Verification items for the finished model (mm, model axes). A direction names the side the tool comes from. Round coordinates to 2 decimals unless told otherwise and drop trailing zeros. Write each loop counter-clockwise with the first axis right and the second up, starting at its lowest first coordinate (ties: lowest second). Pieces come first, ordered by that corner, then holes. Notation, with made-up numbers: (20, -6.5) - (50, -6.5) arc R20 ccw to (50, 21.5) - close; hole circle Ø8 at (67.5, 46). An arc over 180 degrees is marked (long way). Answer as a JSON object with one key per item and string values.
```python
from build123d import *

# Parameters (mm, degrees)
SKETCH2_R                       = 24.765
BOSS_EXTRUDE1_DEPTH             = 10.16
CHAMFER1_SIZE                   = 2.54
CHAMFER2_SIZE                   = 0.254
B_0_238_DIAMETER_HOLE1_D        = 6.0452
B_0_238_DIAMETER_HOLE1_DEPTH    = 3.81
B_0_238_DIAMETER_HOLE1_TIP      = 1.816161307
F_1_4_0_25_DIAMETER_HOLE1_D     = 6.35
F_1_4_0_25_DIAMETER_HOLE1_DEPTH = 7.62
F_1_4_0_25_DIAMETER_HOLE1_TIP   = 1.907732465


with BuildPart() as part:
    # Sketch2 → Boss-Extrude1 (new body)
    with BuildSketch(Plane(origin=(0, 0, 0), x_dir=(1, 0, 0), z_dir=(0, 1, 0))):
        Circle(SKETCH2_R)
    extrude(amount=BOSS_EXTRUDE1_DEPTH)

    # Chamfer1
    chamfer1_edges = [part.edges().sort_by_distance(p)[0] for p in [
        (-24.765, 10.16, 0),
    ]]
    chamfer(chamfer1_edges, length=CHAMFER1_SIZE)

    # Chamfer2
    chamfer2_edges = [part.edges().sort_by_distance(p)[0] for p in [
        (-24.765, 0, 0),
    ]]
    chamfer(chamfer2_edges, length=CHAMFER2_SIZE)

    # B (0.238) Diameter Hole1
    with Locations(Plane(origin=(0, 0, 0), x_dir=(-1, 0, 0), z_dir=(0, -1, 0))):
        with Locations((-4.939140867, 4.939140867), (4.939140867, 4.939140867), (4.939140867, -4.939140867), (-4.939140867, -4.939140867)):
            Hole(B_0_238_DIAMETER_HOLE1_D / 2, depth=B_0_238_DIAMETER_HOLE1_DEPTH)
            with Locations((0, 0, -(B_0_238_DIAMETER_HOLE1_DEPTH + B_0_238_DIAMETER_HOLE1_TIP / 2))):  # 118° drill point
                Cone(0, B_0_238_DIAMETER_HOLE1_D / 2, B_0_238_DIAMETER_HOLE1_TIP, mode=Mode.SUBTRACT)

    # 1/4 (0.25) Diameter Hole1
    with Locations(Plane(origin=(0, 0, 0), x_dir=(-1, 0, 0), z_dir=(0, -1, 0))):
        with Locations((0, 0)):
            Hole(F_1_4_0_25_DIAMETER_HOLE1_D / 2, depth=F_1_4_0_25_DIAMETER_HOLE1_DEPTH)
            with Locations((0, 0, -(F_1_4_0_25_DIAMETER_HOLE1_DEPTH + F_1_4_0_25_DIAMETER_HOLE1_TIP / 2))):  # 118° drill point
                Cone(0, F_1_4_0_25_DIAMETER_HOLE1_D / 2, F_1_4_0_25_DIAMETER_HOLE1_TIP, mode=Mode.SUBTRACT)


solid = part.part
```
Q1. Set-up check for faces 4 (the flat face through (0, 0, 5)), 5 (the cylindrical face through (-7.96, 1.93, 4.81)): record each of +Z, -Z, +X, -X, +Y, -Y from which the full face is reachable in a straight line by a thin tool's end or side.
Geometry check:
{"face 4": "+Z, -Z, +X, -X, -Y", "face 5": "-Y"}
Q2. Gauge pin test, flat ends, axial feed: P1, Ø4, axis at y = 6.5, z = -19.5, coming from the +X side; P2, Ø3.5, axis at x = -4.94, z = -4.94, coming from the -Y side; P3, Ø2, axis at y = 4, z = 4, coming from the -X side. Record the tip position at first contact, or that the pin passes through.
Geometry check:
{"P1": "stops at x = 17.52", "P2": "stops at y = 4.57", "P3": "stops at x = -24.58"}
Q3. Release check for a two-part mould opening along Z. For faces 1 (the conical face through (4.697, 5.311, 5.405)), 2 (the conical face through (21.316, 10.037, -6.713)), 3 (the flat face through (0, 10.16, 0)) record: released by +Z, released by -Z, zero draft, split by the parting line, or undercut.
Geometry check:
{"face 1": "undercut", "face 2": "split by the parting line", "face 3": "zero draft"}
Q4. Material ranges on line 1 along X through (y, z) = (1.75, 3.5); line 2 along Z through (x, y) = (0, 6) (3 decimals), recorded low to high. Write a range as [from, to].
Geometry check:
{"line 1": "x = [-24.52, -7.6], [-2.28, 2.28], [7.6, 24.52]", "line 2": "z = [-24.765, -3.175], [3.175, 24.765]"}
Q5. Section check A-A, the plane y = 2. Record the cut outline in (x, z) (3 decimals), then the cut area to 3 significant figures.
Geometry check:
{"outline": "circle Ø49.53 at (0, 0); hole circle Ø6.045 at (-4.939, -4.939); hole circle Ø6.045 at (-4.939, 4.939); hole circle Ø6.35 at (0, 0); hole circle Ø6.045 at (4.939, -4.939); hole circle Ø6.045 at (4.939, 4.939)", "area": "1,780 mm2"}
